The model under review builds one solid part; all positions refer to its coordinate system, in mm. A direction names the side the tool comes from. Round coordinates to 2 decimals unless told otherwise and drop trailing zeros. Order: outer loops, then holes, each group sorted by start corner. A loop starts at its lowest first (then second) coordinate and runs counter-clockwise, first axis right, second up. Notation, with made-up numbers: M 20,3 L 61,3 A19 ccw 61,32 Z; hole C 63,36 d8. An arc over 180 degrees is marked long. Answer as a JSON object with one key per item and string values. Group by question number.
1) The part is to be moulded in two halves that separate along Z. For faces 1 (the cylindrical face through (-24.85, 8.51, 6.61)), 2 (the flat face through (-15.7, 3.7, 11)), 3 (the flat face through (-6, 22.499, 5)), say which applies: +Z half, -Z half, draft (parallel to the pull), parting line (faces both ways), or undercut.
2) Consider section C-C, the plane z = 3.5. Write out the cut boundary in (x, y).
3) For faces 4 (the cylindrical face through (-24.85, 18.51, 6.61)), 5 (the flat face through (-7.113, 13, 5)), list the 3-axis set-ups (+Z, -Z, +X, -X, +Y, -Y) from which the entire face can be reached by the end or side of a thin tool; tool diameter is ignored.
4) Consider section A-A, the plane y = 21. Write out the cut boundary in (x, z).
5) Consider section D-D, the plane y = 8. Write out the cut boundary in (x, z), then the cut area to 3 significant figures.
6) To check wall thickness, follow line 1 (Y direction, x = -5.9, z = 5.5); line 2 (X direction, y = 15.5, z = 1.25); line 3 (Y direction, x = -20, z = 1). State the ranges of each line that lie inside material, in increasing order.
7) Consider section B-B, the plane z = 5.5. Write out the cut boundary in (x, y).
```python
from build123d import *

# Parameters (mm, degrees)
EXTRUSION1_DEPTH = 11
ESQUISSE3_R      = 1.5
EXTRUSION3_DEPTH = 33.050075964


with BuildPart() as part:
    # Esquisse1 → Extrusion1 (new body)
    with BuildSketch(Plane.XY):
        Polygon((-25.613160064, 22.499052632), (-25.613160064, 2.499052632), (-5.613160064, 2.499052632), (-5.613160064, 22.499052632), (-7.113160064, 22.499052632), (-7.113160064, 3.999052632), (-24.113160064, 3.999052632), (-24.113160064, 22.499052632), align=None)
    extrude(amount=EXTRUSION1_DEPTH)

    # Esquisse3 → Extrusion3 (cut, through all)
    with BuildSketch(Plane(origin=(-5.613160064, 0, 0), x_dir=(0, 0, -1), z_dir=(1, 0, 0))):
        with Locations((-5.5, 7.499052632)):
            Circle(ESQUISSE3_R)
        with Locations((-5.5, 17.499052632)):
            Circle(ESQUISSE3_R)
    extrude(amount=-EXTRUSION3_DEPTH, mode=Mode.SUBTRACT)


solid = part.part
```
Results list:
{
 "1": {"face 1": "undercut", "face 2": "+Z half", "face 3": "draft"},
 "2": {"outline": "M -25.61,2.5 L -5.61,2.5 L -5.61,22.5 L -7.11,22.5 L -7.11,4 L -24.11,4 L -24.11,22.5 L -25.61,22.5 Z"},
 "3": {"face 4": "+X, -X", "face 5": "+Z, -Z, +Y"},
 "4": {"outline": "M -25.61,0 L -24.11,0 L -24.11,11 L -25.61,11 Z; M -7.11,0 L -5.61,0 L -5.61,11 L -7.11,11 Z"},
 "5": {"outline": "M -25.61,0 L -24.11,0 L -24.11,4.09 L -25.61,4.09 Z; M -25.61,6.91 L -24.11,6.91 L -24.11,11 L -25.61,11 Z; M -7.11,0 L -5.61,0 L -5.61,4.09 L -7.11,4.09 Z; M -7.11,6.91 L -5.61,6.91 L -5.61,11 L -7.11,11 Z", "area": "24.5 mm^2"},
 "6": {"line 1": "2.5 to 6, 9 to 16, 19 to 22.5", "line 2": "-25.61 to -24.11, -7.11 to -5.61", "line 3": "2.5 to 4"},
 "7": {"outline": "M -25.61,2.5 L -5.61,2.5 L -5.61,6 L -7.11,6 L -7.11,4 L -24.11,4 L -24.11,6 L -25.61,6 Z; M -25.61,9 L -24.11,9 L -24.11,16 L -25.61,16 Z; M -25.61,19 L -24.11,19 L -24.11,22.5 L -25.61,22.5 Z; M -7.11,9 L -5.61,9 L -5.61,16 L -7.11,16 Z; M -7.11,19 L -5.61,19 L -5.61,22.5 L -7.11,22.5 Z"}
}
